Input: part model. Units: mm. Frame: model coordinates. Round coordinates to 2 decimals unless told otherwise and drop trailing zeros. Loops run counter-clockwise (first coordinate to the right, second up) from the corner with the lowest first, then second, coordinate; pieces in that order, holes last. Notation, with made-up numbers: (16.5, -8.5) -> (53.5, -8.5) arc R25 cw to (53.5, 24.5) -> close; hole circle Ø4 at (9, 88). An arc over 180 degrees is marked (long way). Answer in a Markdown table with one row per item. Add a question column.
Q1. Section A-A, the plane x = -2.5. Output: boundary loops of the cut face in (y, z) (3 decimals), and give its area (3 significant figures).
Q2. Section C-C, the plane y = -1.5. Give the number of separate pieces and of enclosed holes in the cut face, and give its area (3 significant figures).
Q3. Section B-B, the plane z = 0.05. Output: boundary loops of the cut face in (x, y).
Q4. Section D-D, the plane x = 0.5. Output: boundary loops of the cut face in (y, z), and give its area (3 significant figures).
Q5. Ray query, L1, parallel to Y at x = 0.5, z = 1.15; L2, parallel to Y at x = 0, z = 0.7; L3, parallel to Y at x = 5, z = 0.75. Return the intervals inside material, ascending. Write a range as from..to.
```python
from build123d import *

# Parameters (mm, degrees)
SKETCH1_W              = 0.4
SKETCH1_H              = 0.4
BOSS_EXTRUDE1_DEPTH    = 3
BOSS_EXTRUDE1_2_DEPTH  = 3
BOSS_EXTRUDE1_3_DEPTH  = 3
BOSS_EXTRUDE1_4_DEPTH  = 3
BOSS_EXTRUDE1_5_DEPTH  = 3
BOSS_EXTRUDE1_6_DEPTH  = 3
BOSS_EXTRUDE1_7_DEPTH  = 3
BOSS_EXTRUDE1_8_DEPTH  = 3
BOSS_EXTRUDE1_9_DEPTH  = 3
BOSS_EXTRUDE1_10_DEPTH = 3
BOSS_EXTRUDE1_11_DEPTH = 3
BOSS_EXTRUDE1_12_DEPTH = 3
BOSS_EXTRUDE1_13_DEPTH = 3
BOSS_EXTRUDE1_14_DEPTH = 3
SKETCH2_W              = 13.08
SKETCH2_H              = 3
BOSS_EXTRUDE2_DEPTH    = 5
SKETCH3_W              = 9
SKETCH3_H              = 0.64
CUT_EXTRUDE1_DEPTH     = 9.761940424


with BuildPart() as part:
    # Sketch1 → Boss-Extrude1 (new body)
    with BuildSketch(Plane(origin=(0, 0, 0), x_dir=(1, 0, 0), z_dir=(0, 1, 0))):
        with Locations((-2.54, -0.635)):
            Rectangle(SKETCH1_W, SKETCH1_H)
    extrude(amount=-BOSS_EXTRUDE1_DEPTH)



with BuildPart() as body_2:
    # Sketch1 → Boss-Extrude1 2 (new body)
    with BuildSketch(Plane(origin=(0, 0, 0), x_dir=(1, 0, 0), z_dir=(0, 1, 0))):
        with Locations((-3.81, -0.635)):
            Rectangle(SKETCH1_W, SKETCH1_H)
    extrude(amount=-BOSS_EXTRUDE1_2_DEPTH)


with BuildPart() as body_3:
    # Sketch1 → Boss-Extrude1 3 (new body)
    with BuildSketch(Plane(origin=(0, 0, 0), x_dir=(1, 0, 0), z_dir=(0, 1, 0))):
        with Locations((-1.27, -0.635)):
            Rectangle(SKETCH1_W, SKETCH1_H)
    extrude(amount=-BOSS_EXTRUDE1_3_DEPTH)


with BuildPart() as body_4:
    # Sketch1 → Boss-Extrude1 4 (new body)
    with BuildSketch(Plane(origin=(0, 0, 0), x_dir=(1, 0, 0), z_dir=(0, 1, 0))):
        with Locations((0, -0.635)):
            Rectangle(SKETCH1_W, SKETCH1_H)
    extrude(amount=-BOSS_EXTRUDE1_4_DEPTH)


with BuildPart() as body_5:
    # Sketch1 → Boss-Extrude1 5 (new body)
    with BuildSketch(Plane(origin=(0, 0, 0), x_dir=(1, 0, 0), z_dir=(0, 1, 0))):
        with Locations((1.27, -0.635)):
            Rectangle(SKETCH1_W, SKETCH1_H)
    extrude(amount=-BOSS_EXTRUDE1_5_DEPTH)


with BuildPart() as body_6:
    # Sketch1 → Boss-Extrude1 6 (new body)
    with BuildSketch(Plane(origin=(0, 0, 0), x_dir=(1, 0, 0), z_dir=(0, 1, 0))):
        with Locations((2.54, -0.635)):
            Rectangle(SKETCH1_W, SKETCH1_H)
    extrude(amount=-BOSS_EXTRUDE1_6_DEPTH)


with BuildPart() as body_7:
    # Sketch1 → Boss-Extrude1 7 (new body)
    with BuildSketch(Plane(origin=(0, 0, 0), x_dir=(1, 0, 0), z_dir=(0, 1, 0))):
        with Locations((3.81, -0.635)):
            Rectangle(SKETCH1_W, SKETCH1_H)
    extrude(amount=-BOSS_EXTRUDE1_7_DEPTH)


with BuildPart() as body_8:
    # Sketch1 → Boss-Extrude1 8 (new body)
    with BuildSketch(Plane(origin=(0, 0, 0), x_dir=(1, 0, 0), z_dir=(0, 1, 0))):
        with Locations((-2.54, 0.635)):
            Rectangle(SKETCH1_W, SKETCH1_H)
    extrude(amount=-BOSS_EXTRUDE1_8_DEPTH)


with BuildPart() as body_9:
    # Sketch1 → Boss-Extrude1 9 (new body)
    with BuildSketch(Plane(origin=(0, 0, 0), x_dir=(1, 0, 0), z_dir=(0, 1, 0))):
        with Locations((-1.27, 0.635)):
            Rectangle(SKETCH1_W, SKETCH1_H)
    extrude(amount=-BOSS_EXTRUDE1_9_DEPTH)


with BuildPart() as body_10:
    # Sketch1 → Boss-Extrude1 10 (new body)
    with BuildSketch(Plane(origin=(0, 0, 0), x_dir=(1, 0, 0), z_dir=(0, 1, 0))):
        with Locations((0, 0.635)):
            Rectangle(SKETCH1_W, SKETCH1_H)
    extrude(amount=-BOSS_EXTRUDE1_10_DEPTH)


with BuildPart() as body_11:
    # Sketch1 → Boss-Extrude1 11 (new body)
    with BuildSketch(Plane(origin=(0, 0, 0), x_dir=(1, 0, 0), z_dir=(0, 1, 0))):
        with Locations((1.27, 0.635)):
            Rectangle(SKETCH1_W, SKETCH1_H)
    extrude(amount=-BOSS_EXTRUDE1_11_DEPTH)


with BuildPart() as body_12:
    # Sketch1 → Boss-Extrude1 12 (new body)
    with BuildSketch(Plane(origin=(0, 0, 0), x_dir=(1, 0, 0), z_dir=(0, 1, 0))):
        with Locations((2.54, 0.635)):
            Rectangle(SKETCH1_W, SKETCH1_H)
    extrude(amount=-BOSS_EXTRUDE1_12_DEPTH)


with BuildPart() as body_13:
    # Sketch1 → Boss-Extrude1 13 (new body)
    with BuildSketch(Plane(origin=(0, 0, 0), x_dir=(1, 0, 0), z_dir=(0, 1, 0))):
        with Locations((3.81, 0.635)):
            Rectangle(SKETCH1_W, SKETCH1_H)
    extrude(amount=-BOSS_EXTRUDE1_13_DEPTH)


with BuildPart() as body_14:
    # Sketch1 → Boss-Extrude1 14 (new body)
    with BuildSketch(Plane(origin=(0, 0, 0), x_dir=(1, 0, 0), z_dir=(0, 1, 0))):
        with Locations((-3.81, 0.635)):
            Rectangle(SKETCH1_W, SKETCH1_H)
    extrude(amount=-BOSS_EXTRUDE1_14_DEPTH)


with BuildPart() as part_1:
    add(part.part)

    add(body_2.part)  # Boss-Extrude2 merges body 2

    add(body_3.part)  # Boss-Extrude2 merges body 3

    add(body_4.part)  # Boss-Extrude2 merges body 4

    add(body_5.part)  # Boss-Extrude2 merges body 5

    add(body_6.part)  # Boss-Extrude2 merges body 6

    add(body_7.part)  # Boss-Extrude2 merges body 7

    add(body_8.part)  # Boss-Extrude2 merges body 8

    add(body_9.part)  # Boss-Extrude2 merges body 9

    add(body_10.part)  # Boss-Extrude2 merges body 10

    add(body_11.part)  # Boss-Extrude2 merges body 11

    add(body_12.part)  # Boss-Extrude2 merges body 12

    add(body_13.part)  # Boss-Extrude2 merges body 13

    add(body_14.part)  # Boss-Extrude2 merges body 14
    # Sketch2 → Boss-Extrude2 (add)
    with BuildSketch(Plane(origin=(0, 0, 0), x_dir=(1, 0, 0), z_dir=(0, 1, 0))):
        Rectangle(SKETCH2_W, SKETCH2_H)
    extrude(amount=BOSS_EXTRUDE2_DEPTH)

    # Sketch3 → Cut-Extrude1 (cut, through all)
    with BuildSketch(Plane.XY.offset(1.5)):
        with Locations((0, 4.05)):
            Rectangle(SKETCH3_W, SKETCH3_H)
    extrude(amount=-CUT_EXTRUDE1_DEPTH, mode=Mode.SUBTRACT)


solid = part_1.part
```
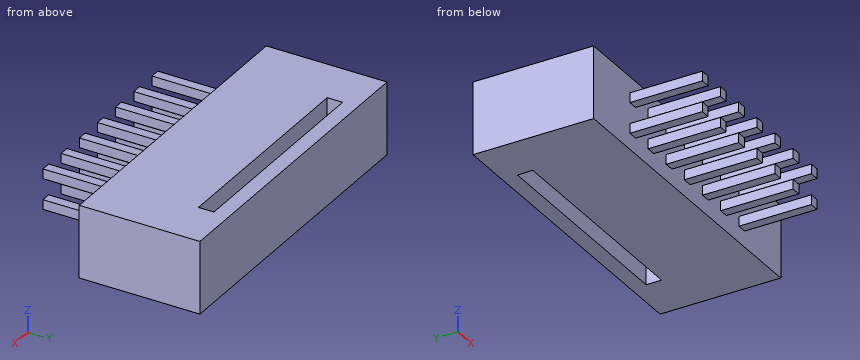
Answer block:
| question | item | result |
|---|---|---|
| 1 | outline | (-3, -0.835) -> (0, -0.835) -> (0, -1.5) -> (3.73, -1.5) -> (3.73, 1.5) -> (0, 1.5) -> (0, 0.835) -> (-3, 0.835) -> (-3, 0.435) -> (0, 0.435) -> (0, -0.435) -> (-3, -0.435) -> close; (4.37, -1.5) -> (5, -1.5) -> (5, 1.5) -> (4.37, 1.5) -> close |
| 1 | area | 15.5 mm^2 |
| 2 | separate pieces | 14 |
| 2 | enclosed holes | 0 |
| 2 | area | 2.24 mm^2 |
| 3 | outline | (-6.54, 0) -> (6.54, 0) -> (6.54, 5) -> (-6.54, 5) -> close; hole (-4.5, 3.73) -> (4.5, 3.73) -> (4.5, 4.37) -> (-4.5, 4.37) -> close |
| 4 | outline | (0, -1.5) -> (3.73, -1.5) -> (3.73, 1.5) -> (0, 1.5) -> close; (4.37, -1.5) -> (5, -1.5) -> (5, 1.5) -> (4.37, 1.5) -> close |
| 4 | area | 13.1 mm^2 |
| 5 | L1 | 0..3.73, 4.37..5 |
| 5 | L2 | -3..3.73, 4.37..5 |
| 5 | L3 | 0..5 |
